Build history of the part. All positions in model axes, mm. A direction names the side the tool comes from. Round coordinates to 2 decimals unless told otherwise and drop trailing zeros. Order: outer loops, then holes, each group sorted by start corner. A loop starts at its lowest first (then second) coordinate and runs counter-clockwise, first axis right, second up. Notation, with made-up numbers: (71.25, 63) -> (124.25, 63) arc R21 ccw to (124.25, 97) -> close; hole circle Ø8 at (73, 43.5). An arc over 180 degrees is marked (long way). Answer as a JSON object with one key per item and string values.
from build123d import *

# Parameters (mm, degrees)
SKETCH_1_R      = 2
EXTRUDE_1_DEPTH = 1.5


with BuildPart() as part:
    # Эскиз1 → Бобышка-Вытянуть1 (new body)
    with BuildSketch(Plane(origin=(0, 0, 0), x_dir=(1, 0, 0), z_dir=(0, 1, 0))):
        with BuildLine():
            Line((3, 0), (31.444558288, 0))
            ThreePointArc((31.444558288, 0), (32.896927043, 0.375), (33.986203609, 1.40625))
            ThreePointArc((33.986203609, 1.40625), (58, -5.5), (33.986203609, -12.40625))
            ThreePointArc((33.986203609, -12.40625), (32.896927043, -11.375), (31.444558288, -11))
            Line((31.444558288, -11), (3, -11))
            ThreePointArc((3, -11), (0.878679656, -10.121320344), (0, -8))
            Line((0, -8), (0, -3))
            ThreePointArc((0, -3), (0.878679656, -0.878679656), (3, 0))
        make_face()
        with Locations((5.5, -5.5)):
            Circle(SKETCH_1_R, mode=Mode.SUBTRACT)
        with Locations((15.5, -5.5)):
            Circle(SKETCH_1_R, mode=Mode.SUBTRACT)
    extrude(amount=EXTRUDE_1_DEPTH)


solid = part.part
1) Pull direction Z, two halves, no side cores. Call faces 3 (the face through (0, 1, 6)), 4 (the face through (13.9, 0.7, 6.7)), 5 (the face through (3.9, 0.7, 6.7)), 6 (the face through (17, 1, 11)): pulls with the +Z half, pulls with the -Z half, needs draft (parallel to the pull), parting line crosses it, or undercut.
Checked values:
{"face 3": "needs draft", "face 4": "undercut", "face 5": "undercut", "face 6": "pulls with the +Z half"}
2) Cut at B-B, the plane z = 5.5. Give the cut face in (x, y), plus the area to 3 significant figures.
Checked values:
{"outline": "(0, 0) -> (3.5, 0) -> (3.5, 1.5) -> (0, 1.5) -> close; (7.5, 0) -> (13.5, 0) -> (13.5, 1.5) -> (7.5, 1.5) -> close; (17.5, 0) -> (58, 0) -> (58, 1.5) -> (17.5, 1.5) -> close", "area": "75.0 mm²"}
3) Cut at D-D, the plane x = 36. Give the cut face in (y, z).
Checked values:
{"outline": "(0, -3.88) -> (1.5, -3.88) -> (1.5, 14.88) -> (0, 14.88) -> close"}
4) Which spindle directions (+Z, -Z, +X, -X, +Y, -Y) get a long thin tool onto all of the face, cutting with end or side? Do faces 1 (the face through (17, 1, 0)), 2 (the face through (36, 1.5, 5)). Say none if no direction does.
Checked values:
{"face 1": "-Z, -X, +Y, -Y", "face 2": "+Z, -Z, +X, -X, +Y"}
5) Cut at A-A, the plane x = 5.5. Give the cut face in (y, z), plus the area to 3 significant figures.
Checked values:
{"outline": "(0, 0) -> (1.5, 0) -> (1.5, 3.5) -> (0, 3.5) -> close; (0, 7.5) -> (1.5, 7.5) -> (1.5, 11) -> (0, 11) -> close", "area": "10.5 mm²"}
6) Probe L1, parallel to X at y = 1.05, z = 5.5; L2, parallel to Z at x = 5.5, y = 1.25; L3, parallel to X at y = 0.7, z = 6.5. List the from-to ranges inside material, lowest first. Write a range as from..to.
Checked values:
{"L1": "x = 0..3.5, 7.5..13.5, 17.5..58", "L2": "z = 0..3.5, 7.5..11", "L3": "x = 0..3.77, 7.23..13.77, 17.23..57.96"}
7) Cut at C-C, the plane y = 0.6. Give the cut face in (x, z), plus the area to 3 significant figures.
Checked values:
{"outline": "(0, 3) arc R3 ccw to (3, 0) -> (31.44, 0) arc R3 cw to (33.99, -1.41) arc R13 ccw (long way) to (33.99, 12.41) arc R3 cw to (31.44, 11) -> (3, 11) arc R3 ccw to (0, 8) -> close; hole circle Ø4 at (5.5, 5.5); hole circle Ø4 at (15.5, 5.5)", "area": "859 mm²"}
